Input: part model. Units: mm. Frame: model coordinates. Give positions to 0.01 mm unless a question says otherwise; leave off trailing zeros. Loops run counter-clockwise (first coordinate to the right, second up) from the corner with the lowest first, then second, coordinate; pieces in that order, holes last.
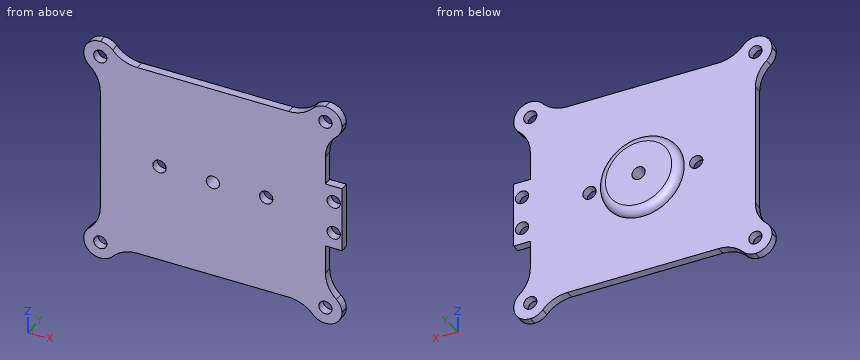
from build123d import *

# Parameters (mm, degrees)
SALIENTE_EXTRUIR1_DEPTH = 5
CROQUIS3_R              = 25
SALIENTE_EXTRUIR2_DEPTH = 5
CORTAR_EXTRUIR1_REACH   = 107.281
CROQUIS4_R              = 4
CORTAR_EXTRUIR2_REACH   = 106.924
CROQUIS5_R              = 4
CORTAR_EXTRUIR8_REACH   = 106.924
CROQUIS12_R             = 4
REDONDEO2_R             = 5


with BuildPart() as part:
    # Croquis1 → Saliente-Extruir1 (new body)
    with BuildSketch(Plane(origin=(0, 0, 0), x_dir=(1, 0, 0), z_dir=(0, 1, 0))):
        with BuildLine():
            Line((78, 60), (78, -60))
            ThreePointArc((78, -60), (75.071067812, -67.071067812), (68, -70))
            Line((68, -70), (-68, -70))
            ThreePointArc((-68, -70), (-75.071067812, -67.071067812), (-78, -60))
            Line((-78, -60), (-78, 60))
            ThreePointArc((-78, 60), (-75.071067812, 67.071067812), (-68, 70))
            Line((-68, 70), (68, 70))
            ThreePointArc((68, 70), (75.071067812, 67.071067812), (78, 60))
        make_face()
    extrude(amount=SALIENTE_EXTRUIR1_DEPTH)

    # Croquis3 → Saliente-Extruir2 (add)
    with BuildSketch(Plane(origin=(0, 5, 0), x_dir=(1, 0, 0), z_dir=(0, 1, 0))):
        with Locations(Location((0, 0, 0), (0, 0, 270))):
            Circle(CROQUIS3_R)
    extrude(amount=SALIENTE_EXTRUIR2_DEPTH)

    # Croquis4 → Cortar-Extruir1 (cut, up to next)
    with BuildSketch(Plane(origin=(0, 10, 0), x_dir=(1, 0, 0), z_dir=(0, 1, 0)), mode=Mode.PRIVATE) as cortar_extruir1_sk1:
        with Locations(Location((0, 0, 0), (0, 0, 270))):
            Circle(CROQUIS4_R)
    cortar_extruir1_tool1 = extrude(cortar_extruir1_sk1.sketch, amount=-CORTAR_EXTRUIR1_REACH, mode=Mode.PRIVATE) & part.part
    add(cortar_extruir1_tool1.solids().sort_by_distance((0, 10, 0))[0], mode=Mode.SUBTRACT)

    # Croquis5 → Cortar-Extruir2 (cut, up to next)
    with BuildSketch(Plane(origin=(0, 5, 0), x_dir=(1, 0, 0), z_dir=(0, 1, 0)), mode=Mode.PRIVATE) as cortar_extruir2_sk1:
        with Locations(Location((-68, -60.171139927, 0), (0, 0, 270))):
            Circle(CROQUIS5_R)
    cortar_extruir2_tool1 = extrude(cortar_extruir2_sk1.sketch, amount=-CORTAR_EXTRUIR2_REACH, mode=Mode.PRIVATE) & part.part
    # Croquis5 → Cortar-Extruir2 (cut, up to next)
    with BuildSketch(Plane(origin=(0, 5, 0), x_dir=(1, 0, 0), z_dir=(0, 1, 0)), mode=Mode.PRIVATE) as cortar_extruir2_sk2:
        with Locations(Location((-68, 59.828860073, 0), (0, 0, 270))):
            Circle(CROQUIS5_R)
    cortar_extruir2_tool2 = extrude(cortar_extruir2_sk2.sketch, amount=-CORTAR_EXTRUIR2_REACH, mode=Mode.PRIVATE) & part.part
    # Croquis5 → Cortar-Extruir2 (cut, up to next)
    with BuildSketch(Plane(origin=(0, 5, 0), x_dir=(1, 0, 0), z_dir=(0, 1, 0)), mode=Mode.PRIVATE) as cortar_extruir2_sk3:
        with Locations(Location((68, -60.171139927, 0), (0, 0, 270))):
            Circle(CROQUIS5_R)
    cortar_extruir2_tool3 = extrude(cortar_extruir2_sk3.sketch, amount=-CORTAR_EXTRUIR2_REACH, mode=Mode.PRIVATE) & part.part
    # Croquis5 → Cortar-Extruir2 (cut, up to next)
    with BuildSketch(Plane(origin=(0, 5, 0), x_dir=(1, 0, 0), z_dir=(0, 1, 0)), mode=Mode.PRIVATE) as cortar_extruir2_sk4:
        with Locations(Location((68, 59.828860073, 0), (0, 0, 270))):
            Circle(CROQUIS5_R)
    cortar_extruir2_tool4 = extrude(cortar_extruir2_sk4.sketch, amount=-CORTAR_EXTRUIR2_REACH, mode=Mode.PRIVATE) & part.part
    # Croquis5 → Cortar-Extruir2 (cut, up to next)
    with BuildSketch(Plane(origin=(0, 5, 0), x_dir=(1, 0, 0), z_dir=(0, 1, 0)), mode=Mode.PRIVATE) as cortar_extruir2_sk5:
        with Locations(Location((32.24, -0.171139927, 0), (0, 0, 270))):
            Circle(CROQUIS5_R)
    cortar_extruir2_tool5 = extrude(cortar_extruir2_sk5.sketch, amount=-CORTAR_EXTRUIR2_REACH, mode=Mode.PRIVATE) & part.part
    # Croquis5 → Cortar-Extruir2 (cut, up to next)
    with BuildSketch(Plane(origin=(0, 5, 0), x_dir=(1, 0, 0), z_dir=(0, 1, 0)), mode=Mode.PRIVATE) as cortar_extruir2_sk6:
        with Locations(Location((-32.24, -0.171139927, 0), (0, 0, 270))):
            Circle(CROQUIS5_R)
    cortar_extruir2_tool6 = extrude(cortar_extruir2_sk6.sketch, amount=-CORTAR_EXTRUIR2_REACH, mode=Mode.PRIVATE) & part.part
    add(cortar_extruir2_tool1.solids().sort_by_distance((-68, 5, 60.17114))[0], mode=Mode.SUBTRACT)
    add(cortar_extruir2_tool2.solids().sort_by_distance((-68, 5, -59.82886))[0], mode=Mode.SUBTRACT)
    add(cortar_extruir2_tool3.solids().sort_by_distance((68, 5, 60.17114))[0], mode=Mode.SUBTRACT)
    add(cortar_extruir2_tool4.solids().sort_by_distance((68, 5, -59.82886))[0], mode=Mode.SUBTRACT)
    add(cortar_extruir2_tool5.solids().sort_by_distance((32.24, 5, 0.17114))[0], mode=Mode.SUBTRACT)
    add(cortar_extruir2_tool6.solids().sort_by_distance((-32.24, 5, 0.17114))[0], mode=Mode.SUBTRACT)

    # Croquis12 → Cortar-Extruir8 (cut, up to next)
    with BuildSketch(Plane(origin=(0, 5, 0), x_dir=(1, 0, 0), z_dir=(0, 1, 0)), mode=Mode.PRIVATE) as cortar_extruir8_sk1:
        with BuildLine():
            Line((68, 70), (-68, 70))
            ThreePointArc((-68, 70), (-63.917517095, 69.128709292), (-60.546440075, 66.666666667))
            ThreePointArc((-60.546440075, 66.666666667), (-53.804286034, 61.742581416), (-45.639320225, 60))
            Line((-45.639320225, 60), (45.639320225, 60))
            ThreePointArc((45.639320225, 60), (53.804286034, 61.742581416), (60.546440075, 66.666666667))
            ThreePointArc((60.546440075, 66.666666667), (63.917517095, 69.128709292), (68, 70))
        make_face()
    cortar_extruir8_tool1 = extrude(cortar_extruir8_sk1.sketch, amount=-CORTAR_EXTRUIR8_REACH, mode=Mode.PRIVATE) & part.part
    # Croquis12 → Cortar-Extruir8 (cut, up to next)
    with BuildSketch(Plane(origin=(0, 5, 0), x_dir=(1, 0, 0), z_dir=(0, 1, 0)), mode=Mode.PRIVATE) as cortar_extruir8_sk2:
        with BuildLine():
            Line((-78, 60), (-78, -60))
            ThreePointArc((-78, -60), (-77.128709292, -55.917517095), (-74.666666667, -52.546440075))
            ThreePointArc((-74.666666667, -52.546440075), (-69.742581416, -45.804286034), (-68, -37.639320225))
            Line((-68, -37.639320225), (-68, 37.639320225))
            ThreePointArc((-68, 37.639320225), (-69.742581416, 45.804286034), (-74.666666667, 52.546440075))
            ThreePointArc((-74.666666667, 52.546440075), (-77.128709292, 55.917517095), (-78, 60))
        make_face()
    cortar_extruir8_tool2 = extrude(cortar_extruir8_sk2.sketch, amount=-CORTAR_EXTRUIR8_REACH, mode=Mode.PRIVATE) & part.part
    # Croquis12 → Cortar-Extruir8 (cut, up to next)
    with BuildSketch(Plane(origin=(0, 5, 0), x_dir=(1, 0, 0), z_dir=(0, 1, 0)), mode=Mode.PRIVATE) as cortar_extruir8_sk3:
        with BuildLine():
            Line((-68, -70), (68, -70))
            ThreePointArc((68, -70), (63.917517095, -69.128709292), (60.546440075, -66.666666667))
            ThreePointArc((60.546440075, -66.666666667), (53.804286034, -61.742581416), (45.639320225, -60))
            Line((45.639320225, -60), (-45.639320225, -60))
            ThreePointArc((-45.639320225, -60), (-53.804286034, -61.742581416), (-60.546440075, -66.666666667))
            ThreePointArc((-60.546440075, -66.666666667), (-63.917517095, -69.128709292), (-68, -70))
        make_face()
    cortar_extruir8_tool3 = extrude(cortar_extruir8_sk3.sketch, amount=-CORTAR_EXTRUIR8_REACH, mode=Mode.PRIVATE) & part.part
    # Croquis12 → Cortar-Extruir8 (cut, up to next)
    with BuildSketch(Plane(origin=(0, 5, 0), x_dir=(1, 0, 0), z_dir=(0, 1, 0)), mode=Mode.PRIVATE) as cortar_extruir8_sk4:
        with BuildLine():
            ThreePointArc((74.666666667, -52.546440075), (77.128709292, -55.917517095), (78, -60))
            Line((78, -60), (78, -20))
            Line((78, -20), (68, -20))
            Line((68, -20), (68, -37.639320225))
            ThreePointArc((68, -37.639320225), (69.742581416, -45.804286034), (74.666666667, -52.546440075))
        make_face()
    cortar_extruir8_tool4 = extrude(cortar_extruir8_sk4.sketch, amount=-CORTAR_EXTRUIR8_REACH, mode=Mode.PRIVATE) & part.part
    # Croquis12 → Cortar-Extruir8 (cut, up to next)
    with BuildSketch(Plane(origin=(0, 5, 0), x_dir=(1, 0, 0), z_dir=(0, 1, 0)), mode=Mode.PRIVATE) as cortar_extruir8_sk5:
        with BuildLine():
            Line((68, 20), (78, 20))
            Line((78, 20), (78, 60))
            ThreePointArc((78, 60), (77.128709292, 55.917517095), (74.666666667, 52.546440075))
            ThreePointArc((74.666666667, 52.546440075), (69.742581416, 45.804286034), (68, 37.639320225))
            Line((68, 37.639320225), (68, 20))
        make_face()
    cortar_extruir8_tool5 = extrude(cortar_extruir8_sk5.sketch, amount=-CORTAR_EXTRUIR8_REACH, mode=Mode.PRIVATE) & part.part
    # Croquis12 → Cortar-Extruir8 (cut, up to next)
    with BuildSketch(Plane(origin=(0, 5, 0), x_dir=(1, 0, 0), z_dir=(0, 1, 0)), mode=Mode.PRIVATE) as cortar_extruir8_sk6:
        with Locations(Location((73, 10, 0), (0, 0, 270))):
            Circle(CROQUIS12_R)
    cortar_extruir8_tool6 = extrude(cortar_extruir8_sk6.sketch, amount=-CORTAR_EXTRUIR8_REACH, mode=Mode.PRIVATE) & part.part
    # Croquis12 → Cortar-Extruir8 (cut, up to next)
    with BuildSketch(Plane(origin=(0, 5, 0), x_dir=(1, 0, 0), z_dir=(0, 1, 0)), mode=Mode.PRIVATE) as cortar_extruir8_sk7:
        with Locations(Location((73, -10, 0), (0, 0, 270))):
            Circle(CROQUIS12_R)
    cortar_extruir8_tool7 = extrude(cortar_extruir8_sk7.sketch, amount=-CORTAR_EXTRUIR8_REACH, mode=Mode.PRIVATE) & part.part
    add(cortar_extruir8_tool1.solids().sort_by_distance((0, 5, -65.214104))[0], mode=Mode.SUBTRACT)
    add(cortar_extruir8_tool2.solids().sort_by_distance((-73.248187, 5, 0))[0], mode=Mode.SUBTRACT)
    add(cortar_extruir8_tool3.solids().sort_by_distance((0, 5, 65.214104))[0], mode=Mode.SUBTRACT)
    add(cortar_extruir8_tool4.solids().sort_by_distance((73.412248, 5, 35.448838))[0], mode=Mode.SUBTRACT)
    add(cortar_extruir8_tool5.solids().sort_by_distance((73.412248, 5, -35.448838))[0], mode=Mode.SUBTRACT)
    add(cortar_extruir8_tool6.solids().sort_by_distance((73, 5, -10))[0], mode=Mode.SUBTRACT)
    add(cortar_extruir8_tool7.solids().sort_by_distance((73, 5, 10))[0], mode=Mode.SUBTRACT)

    # Redondeo2
    redondeo2_edges = [part.edges().sort_by_distance(p)[0] for p in [
        (0, 10, -25),
    ]]
    fillet(redondeo2_edges, radius=REDONDEO2_R - 0.0001)  # a hair under: the kernel refuses the full size


solid = part.part
(1) Cut plane C-C (y = 3). Count the separate pieces of the cut face and the enclosed holes in it, and give its area (3 significant figures).
Values follow:
separate pieces: 1
enclosed holes: 9
area: 17,400 mm2
(2) Cut plane B-B (x = -32.24). Return the cut outline in (y, z), and give its area (3 significant figures).
Values follow:
outline: (0, -60) - (5, -60) - (5, -3.83) - (0, -3.83) - close; (0, 4.17) - (5, 4.17) - (5, 60) - (0, 60) - close
area: 560 mm2
(3) Cut plane D-D (x = 34). Return the cut outline in (y, z).
Values follow:
outline: (0, -60) - (5, -60) - (5, -3.42) - (0, -3.42) - close; (0, 3.76) - (5, 3.76) - (5, 60) - (0, 60) - close
(4) Ray query, probe 1 along Y at (x, z) = (-4, 27); probe 2 along X at (y, z) = (4.25, 29); probe 3 along Z at (x, y) = (21.5, 1). Return the intervals inside material, ascending.
Values follow:
probe 1: y = 0 to 5
probe 2: x = -68 to 68
probe 3: z = -60 to 60
(5) Pin query (flat end, axial travel): pin 1 Ø13 at (x, z) = (73, -10) entering from +Y; pin 2 Ø2.5 at (x, y) = (75, 2.5) entering from -Z; pin 3 Ø1.5 at (y, z) = (2, -26.5) entering from +X; pin 4 Ø10.5 at (x, z) = (0, 0) entering from +Y. Return the tip coordinate at first contact, or that it passes through.
Values follow:
pin 1: stops at y = 5
pin 2: stops at z = -68.18
pin 3: stops at x = 68
pin 4: stops at y = 10
